```python
from build123d import *

# Parameters (mm, degrees)
TORUS_R                 = 0.3
TORUS_ANGLE             = 90
TORUS_ROLL_ANGLE        = -90
TORUS001_R              = 0.3
TORUS001_ANGLE          = 90
CYLINDER008_R           = 0.3
CYLINDER008_DEPTH       = 11
CYLINDER008_PITCH_ANGLE = -90


with BuildPart() as torus:
    # Torus → Torus (revolve)
    with BuildSketch(Plane.XZ):
        with Locations((5, 0)):
            Circle(TORUS_R)
    revolve(axis=Axis((0, 0, 0), (0, 0, 1)), revolution_arc=TORUS_ANGLE)


with BuildPart() as torus_1:
    # Torus roll: moved
    add(torus.part.rotate(Axis((0, 0, 0), (1, 0, 0)), TORUS_ROLL_ANGLE))


with BuildPart() as torus_2:
    # Torus placement: moved
    add(torus_1.part.moved(Location((7.3, -2.7, 12))))


with BuildPart() as cone001:
    # Cone001 → Cone001 (revolve)
    with BuildSketch(Plane(origin=(12.2, -2.6, 11.8), x_dir=(1, 0, 0), z_dir=(0, -1, 0))):
        Polygon((0, 0), (1, 0), (0, 2), align=None)
    revolve(axis=Axis((12.2, -2.6, 11.8), (0, 0, 1)))


with BuildPart() as cone:
    # Cone → Cone (revolve)
    with BuildSketch(Plane(origin=(12.3, -2.6, 0), x_dir=(1, 0, 0), z_dir=(0, -1, 0))):
        Polygon((0, 0), (1, 2), (0, 2), align=None)
    revolve(axis=Axis((12.3, -2.6, 0), (0, 0, 1)))


with BuildPart() as torus001:
    # Torus001 → Torus001 (revolve)
    with BuildSketch(Plane(origin=(7.3, -2.7, 2), x_dir=(0, 0, 1), z_dir=(-1, 0, 0))):
        with Locations((5, 0)):
            Circle(TORUS001_R)
    revolve(axis=Axis((7.3, -2.7, 2), (0, 1, 0)), revolution_arc=TORUS001_ANGLE)


with BuildPart() as fusion012:
    # Cylinder008 → Cylinder008 (new body)
    with BuildSketch(Plane.XY):
        Circle(CYLINDER008_R)
    extrude(amount=CYLINDER008_DEPTH)


with BuildPart() as fusion012_1:
    # Cylinder008 pitch: moved
    add(fusion012.part.rotate(Axis((0, 0, 0), (0, 1, 0)), CYLINDER008_PITCH_ANGLE))


with BuildPart() as fusion012_2:
    # Cylinder008 placement: moved
    add(fusion012_1.part.moved(Location((7.3, -2.7, 7))))

    # Fusion012: union Torus, Cone001, Cone, Torus001
    add(torus_2.part)
    add(cone001.part)
    add(cone.part)
    add(torus001.part)


with BuildPart() as fusion012_3:
    # Fusion012 placement: moved
    add(fusion012_2.part.moved(Location((0, 0, -2.36))))


solid = fusion012_3.part
```
Model file for the job. Use its own axes, mm. Coordinates: 2 decimals unless noted, no trailing zeros. Loops run counter-clockwise (first coordinate to the right, second up) from the corner with the lowest first, then second, coordinate; pieces in that order, holes last. Notation, with made-up numbers: (-38.5, 6) -> (19.5, 6) arc R22 cw to (19.5, 42) -> close; hole circle Ø10 at (-19, 46.5). An arc over 180 degrees is marked (long way). Answer as a JSON object with one key per item and string values.
Q1. Probe probe 1 along X at (y, z) = (-2.95, 9.25); probe 2 along Z at (x, y) = (-0.5, -2.85); probe 3 along X at (y, z) = (-2.45, -1). List the from-to ranges inside material, lowest first.
Report:
{"probe 1": "x = 12.12 to 12.45", "probe 2": "z = 4.38 to 4.9", "probe 3": "x = 11.64 to 12.96"}
Q2. Pull direction Z, two halves, no side cores. Call faces 1 (the conical face through (12.666, -2.752, -1.568)), 2 (the conical face through (12.55, -2.75, 10.68)), 3 (the flat face through (12, -2, 9.44)): released by +Z, released by -Z, zero draft, split by the parting line, or undercut.
Report:
{"face 1": "released by -Z", "face 2": "released by +Z", "face 3": "undercut"}
Q3. Cut at B-B (z = -1). List the corners of the cut face in (x, y), and give its area (3 significant figures).
Report:
{"outline": "circle Ø1.36 at (12.3, -2.6)", "area": "1.45 mm2"}
Q4. Cut at A-A (x = 2.25). List the corners of the cut face in (y, z), and give its area (3 significant figures).
Report:
{"outline": "circle Ø0.6 at (-2.7, 4.64)", "area": "0.283 mm2"}
Q5. Flat gauge pins, fed straight in: P1, Ø0.6, axis at x = 12, y = -2, coming from the -Z side; P2, Ø1.5, axis at x = 11.5, z = 3, coming from the +Y side. Where does each tip first touch, or does it go through?
Report:
{"P1": "stops at z = -1.62", "P2": "stops at y = -2.4"}
